CAD build for the part. Positions are in the model's coordinates, mm. Face numbers are marked on the shaded views. A direction names the side the tool comes from. Coordinates: 2 decimals unless noted, no trailing zeros. Order: outer loops, then holes, each group sorted by start corner. A loop starts at its lowest first (then second) coordinate and runs counter-clockwise, first axis right, second up. Notation, with made-up numbers: (-24, 72.25) - (0, 72.25) arc R28 ccw to (0, 90.25) - close; hole circle Ø3 at (37, 86.5). An arc over 180 degrees is marked (long way). Return JSON: item names as keys, results as strings.
from build123d import *

# Parameters (mm, degrees)
SKETCH_1_W      = 30
SKETCH_1_H      = 30
SKETCH_1_R      = 13.5
EXTRUDE_1_DEPTH = 10
EXTRUDE_2_DEPTH = 1
EXTRUDE_3_DEPTH = 7


with BuildPart() as part:
    # 草图1 → 凸台-拉伸1 (new body)
    with BuildSketch(Plane.XY):
        with Locations((-25.822727996, 31.492551329)):
            Rectangle(SKETCH_1_W, SKETCH_1_H)
        with Locations((-25.822727996, 31.492551329)):
            Circle(SKETCH_1_R, mode=Mode.SUBTRACT)
    extrude(amount=EXTRUDE_1_DEPTH)

    # 草图2 → 凸台-拉伸2 (add)
    with BuildSketch(Plane.XY.offset(10)):
        Polygon((-32.397789449, 44.701032769), (-24.966802837, 33.924156896), (-11.116377527, 33.924156896), (-11.116377527, 32.134495199), (-23.682915097, 32.134495199), (-32.397789449, 18.361881267), (-34.074436385, 19.422810401), (-25.822727996, 31.492551329), (-34.373088606, 43.892812528), (-32.550272533, 45.149700145), align=None)
    extrude(amount=-EXTRUDE_2_DEPTH)

    # 草图3 → 凸台-拉伸3 (add)
    with BuildSketch(Plane(origin=(0, 0, 9), x_dir=(-1, 0, 0), z_dir=(0, 0, -1))):
        Polygon((22.515744425, 34.818987745), (18.780798274, 41.082803685), (25.822727996, 44.428692946), (27.690201072, 35.402573081), (27.690201072, 33.583732117), (29.149164412, 34.7995349), (35.412980353, 38.534481051), (38.758869613, 31.492551329), (29.732749748, 29.625078253), (27.913908784, 29.625078253), (29.129711567, 28.166114913), (32.864657718, 21.902298973), (25.822727996, 18.556409712), (23.955254921, 27.582529577), (23.955254921, 29.401370541), (22.49629158, 28.185567758), (16.23247564, 24.450621607), (12.886586379, 31.492551329), (21.912706244, 33.360024404), (23.731547209, 33.360024404), align=None)
    extrude(amount=EXTRUDE_3_DEPTH)


solid = part.part
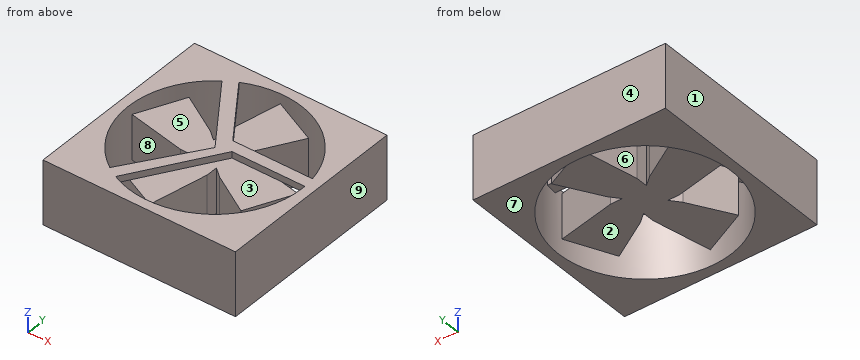
Item 1: Mould opens along X. For the marked faces 1, 2, 3 and 4 say: released by +X, released by -X, zero draft, split by the parting line, or undercut.
Findings below:
{"face 1": "released by -X", "face 2": "undercut", "face 3": "undercut", "face 4": "zero draft"}
Item 2: Band-saw the part on D-D, the plane z = 1.25. List the corners of the cut face in (x, y), then the cut area to 3 significant figures.
Findings below:
{"outline": "(-40.82, 16.49) - (-10.82, 16.49) - (-10.82, 46.49) - (-40.82, 46.49) - close; hole circle Ø27 at (-25.82, 31.49)", "area": "327 mm²"}
Item 3: Band-saw the part on A-A, the plane z = 4. List the corners of the cut face in (x, y), then the cut area to 3 significant figures.
Findings below:
{"outline": "(-40.82, 16.49) - (-10.82, 16.49) - (-10.82, 46.49) - (-40.82, 46.49) - close; (-38.76, 31.49) - (-29.73, 29.63) - (-27.91, 29.63) - (-29.13, 28.17) - (-32.86, 21.9) - (-25.82, 18.56) - (-23.96, 27.58) - (-23.96, 29.4) - (-22.5, 28.19) - (-16.23, 24.45) - (-12.89, 31.49) - (-21.91, 33.36) - (-23.73, 33.36) - (-22.52, 34.82) - (-18.78, 41.08) - (-25.82, 44.43) - (-27.69, 35.4) - (-27.69, 33.58) - (-29.15, 34.8) - (-35.41, 38.53) - close; hole circle Ø27 at (-25.82, 31.49)", "area": "583 mm²"}
Item 4: Band-saw the part on B-B, the plane x = -37.5. List the corners of the cut face in (y, z).
Findings below:
{"outline": "(16.49, 0) - (24.72, 0) - (24.72, 10) - (16.49, 10) - close; (31.23, 2) - (34.14, 2) - (34.14, 9) - (31.23, 9) - close; (38.27, 0) - (46.49, 0) - (46.49, 10) - (38.27, 10) - close"}
Item 5: Drop flat-ended pins along their axis: P1, Ø4, axis at x = -22, y = 28, coming from the +Z side; P2, Ø5, axis at x = -27, y = 30.5, coming from the -Z side; P3, Ø1.9, axis at x = -30.5, y = 38, coming from the -Z side. Give the stop position or say it passes through.
Findings below:
{"P1": "stops at z = 9", "P2": "stops at z = 2", "P3": "stops at z = 9"}
Item 6: Band-saw the part on C-C, the plane y = 31. List the corners of the cut face in (x, z), then the cut area to 3 significant figures.
Findings below:
{"outline": "(-40.82, 0) - (-39.31, 0) - (-39.31, 10) - (-40.82, 10) - close; (-36.38, 2) - (-13.12, 2) - (-13.12, 9) - (-24.4, 9) - (-24.4, 10) - (-26.16, 10) - (-26.16, 9) - (-36.38, 9) - close; (-12.33, 0) - (-10.82, 0) - (-10.82, 10) - (-12.33, 10) - close", "area": "195 mm²"}
Item 7: Wall check: L1, parallel to X at y = 21.25, z = 7; L2, parallel to Y at x = -23.5, z = 6; L3, parallel to Y at x = -14.25, z = 3.75. Give the ranges that are in metal, low to high. Write a range as [from, to].
Findings below:
{"L1": "x = [-40.82, -34.62], [-31.49, -25.27], [-17.03, -10.82]", "L2": "y = [16.49, 18.19], [29.02, 33.36], [33.64, 43.33], [44.79, 46.49]", "L3": "y = [16.49, 24.54], [28.62, 31.77], [38.44, 46.49]"}
Item 8: Which spindle directions (+Z, -Z, +X, -X, +Y, -Y) get a long thin tool onto all of the face, cutting with end or side? Do the marked faces 5, 6, 7, 8 and 9. Say none if no direction does.
Findings below:
{"face 5": "+Z", "face 6": "-Z", "face 7": "-Z, +X, -X, +Y, -Y", "face 8": "+Z, -Z", "face 9": "+Z, -Z, +X, +Y, -Y"}
